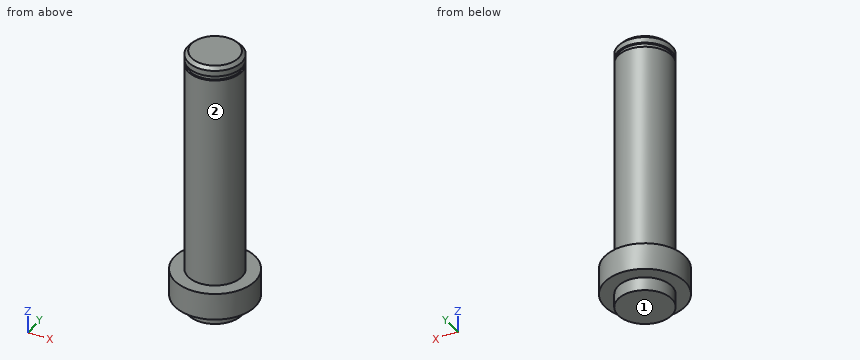
Autodesk Inventor part; units mm, degrees
ref_plane "YZ Plane" through (0, 0, 0) normal (1, 0, 0) x (0, 1, 0)
ref_plane "XZ Plane" through (0, 0, 0) normal (0, 1, 0) x (-1, 0, 0)
ref_plane "XY Plane" through (0, 0, 0) normal (0, 0, 1) x (1, 0, 0)
sketch "Sketch1" plane through (0, 0, 0) normal (0, 0, 1) x (1, 0, 0)
  circle A0 centre (0, 0) radius 9.525
  dimension "d0" = 19.05
extrude "Extrusion1" add sketch "Sketch1" along normal blind 6.35
sketch "Sketch2" plane through (0, 0, 6.35) normal (0, 0, 1) x (1, 0, 0)
  circle A0 centre (0, 0) radius 6.35
  dimension "d3" = 12.7
extrude "Extrusion2" add sketch "Sketch2" along normal blind 50.8
sketch "Sketch3" plane through (0, 0, 57.15) normal (0, 0, 1) x (1, 0, 0)
  circle A0 centre (0, 0) radius 5.9531
  dimension "d6" = 11.9062
extrude "Extrusion3" add sketch "Sketch3" along normal blind 1.016
sketch "Sketch4" plane through (0, 0, 58.166) normal (0, 0, 1) x (1, 0, 0)
  circle A0 centre (0, 0) radius 6.35
extrude "Extrusion4" add sketch "Sketch4" along normal blind 2.159
chamfer "Chamfer1" distance 0.7937 angle 45 1 edges at (-6.35, 0, 60.325)
sketch "Sketch5" plane through (0, 0, 0) normal (0, 0, -1) x (-1, 0, 0)
  circle A0 centre (0, 0) radius 6.35
  dimension "d14" = 12.7
extrude "Extrusion5" add sketch "Sketch5" along normal blind 3.175
properties part number "A1-18002-100-38 Leg hinge pin" material "Steel, Mild"
Work out the finished part from the listing and answer in its coordinate system (mm). Face numbers are marked on the shaded views. A direction names the side the tool comes from. Give positions to 0.01 mm unless a question says otherwise; leave off trailing zeros. Order: outer loops, then holes, each group sorted by start corner. A loop starts at its lowest first (then second) coordinate and runs counter-clockwise, first axis right, second up. Notation, with made-up numbers: (43.25, 33.5) - (59.25, 33.5) arc R12 ccw to (59.25, 53.5) - close; hole circle Ø5 at (24.25, 1). An arc over 180 degrees is marked (long way). One line per item, written item: value. Start each with the question number.
1. Section D-D, the plane x = -8 is taken. Write down the section's boundary in (y, z), then the cut area to 3 significant figures.
2. Section A-A, the plane x = 0 is taken. Write down the section's boundary in (y, z) (3 decimals).
3. Consider line 1 (Z direction, x = -1.25, y = 7.5); line 2 (Z direction, x = 5, y = -3.5) (3 decimals); line 3 (Y direction, x = 1, z = 46.5). Determine where each line is inside the solid, lowest interval first.
4. Each of these flat-tipped pins is pushed along its axis until it touches: pin 1 Ø3 at (y, z) = (-2, 24) entering from +X; pin 2 Ø2 at (x, z) = (6, 13) entering from -Y; pin 3 Ø10 at (x, z) = (-4.5, 53) entering from -Y. Where does it stop, or does it pass through?
5. Section C-C, the plane z = 9 is taken. Write down the section's boundary in (x, y).
6. Which of the six approach directions +Z, -Z, +X, -X, +Y, -Y give full straight-line access (tool end or side, diameter ignored) to the marked faces 1 and 2?
Filled sheet:
1. outline: (-5.17, 0) - (5.17, 0) - (5.17, 6.35) - (-5.17, 6.35) - close
1. area: 65.7 mm²
2. outline: (-9.525, 0) - (-6.35, 0) - (-6.35, -3.175) - (6.35, -3.175) - (6.35, 0) - (9.525, 0) - (9.525, 6.35) - (6.35, 6.35) - (6.35, 57.15) - (5.953, 57.15) - (5.953, 58.166) - (6.35, 58.166) - (6.35, 59.531) - (5.556, 60.325) - (-5.556, 60.325) - (-6.35, 59.531) - (-6.35, 58.166) - (-5.953, 58.166) - (-5.953, 57.15) - (-6.35, 57.15) - (-6.35, 6.35) - (-9.525, 6.35) - close
3. line 1: 0 to 6.35
3. line 2: -3.175 to 57.15, 58.166 to 59.778
3. line 3: -6.27 to 6.27
4. pin 1: x = 6.33
4. pin 2: y = -3.91
4. pin 3: y = -6.35
5. outline: circle Ø12.7 at (0, 0)
6. face 1: -Z, +X, -X, +Y, -Y
6. face 2: +Z
